Work out the finished part from the listing and answer in its coordinate system (mm). A direction names the side the tool comes from. Round coordinates to 2 decimals unless told otherwise and drop trailing zeros. Write each loop counter-clockwise with the first axis right and the second up, starting at its lowest first coordinate (ties: lowest second). Pieces come first, ordered by that corner, then holes. Notation, with made-up numbers: M -31,-26.75 L 19,-26.75 A15 ccw 19,2.25 Z; hole C 70,-21.5 d10. An arc over 180 degrees is marked long. One line per item, written item: value. Start each with the question number.
Q1. Find section A-A (z = 6). Write down the section's boundary in (x, y).
Q2. Consider probe 1 along Y at (x, z) = (387, -2); probe 2 along Z at (x, y) = (413, -11). Determine where each line is inside the solid, lowest interval first.
Q3. The mould has two halves that part along Y. Classify faces 3 (the flat face through (376, -2, -28.181)), 4 (the flat face through (376, -2, 20.079)), 5 (the flat face through (376, -14.7, -5)): released by +Y, released by -Y, zero draft, split by the parting line, or undercut.
Q4. A tool of negligible diameter and unlimited length cuts with its end or side. For faces 1 (the flat face through (376, 8.16, -5)), 2 (the flat face through (762, 8.4, -5.2)), from which of +Z, -Z, +X, -X, +Y, -Y can it reach the whole face along a straight path? Write none if from no direction.
Q5. Given pin 1 Ø8 at (x, y) = (315.78, -2) entering from -Z, flat-ended and moving along its own axis, determine where the tip first touches the part or whether it passes through.
from build123d import *

# Parameters (mm, degrees)
SKETCH3_W           = 50.8
SKETCH3_H           = 25.4
SKETCH3_W_2         = 45.72
SKETCH3_H_2         = 20.32
BOSS_EXTRUDE1_DEPTH = 762
SKETCH5_R           = 5.08
CUT_EXTRUDE2_DEPTH  = 127
SKETCH5_8_R         = 5.08
CUT_EXTRUDE5_DEPTH  = 127
SKETCH5_9_R         = 5.08
CUT_EXTRUDE6_DEPTH  = 127


with BuildPart() as part:
    # Sketch3 → Boss-Extrude1 (new body)
    with BuildSketch(Plane(origin=(0, 0, 0), x_dir=(0, 0, -1), z_dir=(1, 0, 0))):
        with Locations((5.321216632, -1.999606833)):
            Rectangle(SKETCH3_W, SKETCH3_H)
        with Locations((5.321216632, -1.999606833)):
            Rectangle(SKETCH3_W_2, SKETCH3_H_2, mode=Mode.SUBTRACT)
    extrude(amount=BOSS_EXTRUDE1_DEPTH)

    # Sketch5 → Cut-Extrude2 (cut)
    with BuildSketch(Plane.XY.offset(20.078783368)):
        with Locations((10.978833808, -1.999606833)):
            Circle(SKETCH5_R)
        with Locations((36.378833808, -1.999606833)):
            Circle(SKETCH5_R)
        with Locations((61.778833808, -1.999606833)):
            Circle(SKETCH5_R)
        with Locations((87.178833808, -1.999606833)):
            Circle(SKETCH5_R)
        with Locations((112.578833808, -1.999606833)):
            Circle(SKETCH5_R)
        with Locations((137.978833808, -1.999606833)):
            Circle(SKETCH5_R)
        with Locations((163.378833808, -1.999606833)):
            Circle(SKETCH5_R)
        with Locations((188.778833808, -1.999606833)):
            Circle(SKETCH5_R)
        with Locations((214.178833808, -1.999606833)):
            Circle(SKETCH5_R)
        with Locations((239.578833808, -1.999606833)):
            Circle(SKETCH5_R)
        with Locations((264.978833808, -1.999606833)):
            Circle(SKETCH5_R)
        with Locations((290.378833808, -1.999606833)):
            Circle(SKETCH5_R)
        with Locations((315.778833808, -1.999606833)):
            Circle(SKETCH5_R)
        with Locations((341.178833808, -1.999606833)):
            Circle(SKETCH5_R)
        with Locations((366.578833808, -1.999606833)):
            Circle(SKETCH5_R)
        with Locations((391.978833808, -1.999606833)):
            Circle(SKETCH5_R)
        with Locations((417.378833808, -1.999606833)):
            Circle(SKETCH5_R)
        with Locations((442.778833808, -1.999606833)):
            Circle(SKETCH5_R)
        with Locations((468.178833808, -1.999606833)):
            Circle(SKETCH5_R)
        with Locations((493.578833808, -1.999606833)):
            Circle(SKETCH5_R)
        with Locations((518.978833808, -1.999606833)):
            Circle(SKETCH5_R)
        with Locations((544.378833808, -1.999606833)):
            Circle(SKETCH5_R)
        with Locations((569.778833808, -1.999606833)):
            Circle(SKETCH5_R)
        with Locations((595.178833808, -1.999606833)):
            Circle(SKETCH5_R)
        with Locations((620.578833808, -1.999606833)):
            Circle(SKETCH5_R)
        with Locations((645.978833808, -1.999606833)):
            Circle(SKETCH5_R)
        with Locations((671.378833808, -1.999606833)):
            Circle(SKETCH5_R)
        with Locations((696.778833808, -1.999606833)):
            Circle(SKETCH5_R)
    extrude(amount=-CUT_EXTRUDE2_DEPTH, mode=Mode.SUBTRACT)

    # Sketch5<8> → Cut-Extrude5 (cut)
    with BuildSketch(Plane.XY.offset(20.078783368)):
        with Locations((722.178833808, -1.999606833)):
            Circle(SKETCH5_8_R)
    extrude(amount=-CUT_EXTRUDE5_DEPTH, mode=Mode.SUBTRACT)

    # Sketch5<9> → Cut-Extrude6 (cut)
    with BuildSketch(Plane.XY.offset(20.078783368)):
        with Locations((747.578833808, -1.999606833)):
            Circle(SKETCH5_9_R)
    extrude(amount=-CUT_EXTRUDE6_DEPTH, mode=Mode.SUBTRACT)


solid = part.part
The answers:
1. outline: M 0,-14.7 L 762,-14.7 L 762,-12.16 L 0,-12.16 Z; M 0,8.16 L 762,8.16 L 762,10.7 L 0,10.7 Z
2. probe 1: -14.7 to -12.16, 8.16 to 10.7
2. probe 2: -30.72 to -28.18, 17.54 to 20.08
3. face 3: undercut
3. face 4: zero draft
3. face 5: released by -Y
4. face 1: +X, -X
4. face 2: +Z, -Z, +X, +Y, -Y
5. pin 1: through
